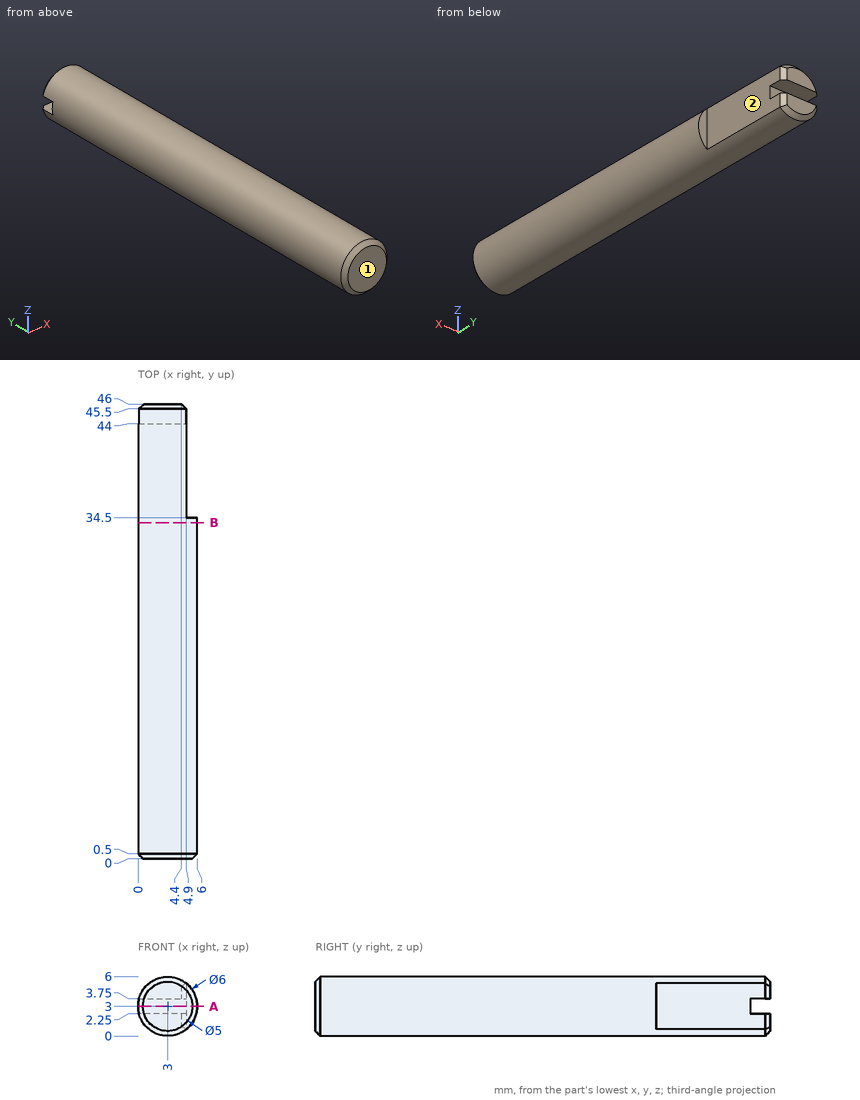
Check sheet for the drawn part. Datum: minimum x, y, z corner. Units: mm. A direction names the side the tool comes from. Give positions to 0.01 mm unless a question says otherwise; leave off trailing zeros. Loops run counter-clockwise (first coordinate to the right, second up) from the corner with the lowest first, then second, coordinate; pieces in that order, holes last. Notation, with made-up numbers: M 32.5,11 L 89.5,11 A8 ccw 89.5,18 Z; hole C 73.25,30.5 d3. An arc over 180 degrees is marked long. Answer as CSV lines item,"result".
Item 1: Set-up check for the marked faces 1 and 2: record each of +Z, -Z, +X, -X, +Y, -Y from which the full face is reachable in a straight line by a thin tool's end or side.
Reply:
face 1,"+Z, -Z, +X, -X, -Y"
face 2,"+Z, -Z, +X, +Y"
Item 2: Scan lines: L1, parallel to Y at x = 5, z = 3; L2, parallel to Z at x = 3.1, y = 36; L3, parallel to Y at x = 2.7, z = 2.8. Record each from-to range of solid material in increasing order.
Reply:
L1,"0 to 34.5"
L2,"0 to 6"
L3,"0 to 44"
Item 3: Sectioned sample at A-A, the plane z = 3. Enter the section's corners in (x, y).
Reply:
outline,"M 0,0.5 L 0.5,0 L 5.5,0 L 6,0.5 L 6,34.5 L 4.9,34.5 L 4.9,44 L 0,44 Z"
Item 4: Sectioned sample at B-B, the plane y = 34. Enter the section's corners in (x, z).
Reply:
outline,"C 3,3 d6"
Item 5: Depth check by flat-ended pin: pin 1 Ø2 at (y, z) = (7, 5.5) entering from -X; pin 2 Ø1.5 at (y, z) = (40, 2) entering from +X; pin 3 Ø0.6 at (x, y) = (2.5, 45.5) entering from +Z. Enter the tip coordinate at first touch or a pass-through.
Reply:
pin 1,"x = 0.4"
pin 2,"x = 4.9"
pin 3,"z = 5.99"
